CAD build for the part. Positions are in the model's coordinates, mm. A direction names the side the tool comes from. Round coordinates to 2 decimals unless told otherwise and drop trailing zeros. Write each loop counter-clockwise with the first axis right and the second up, starting at its lowest first coordinate (ties: lowest second). Pieces come first, ordered by that corner, then holes. Notation, with made-up numbers: (2, -3.75) - (23, -3.75) arc R17 cw to (23, 1.25) - close; hole circle Ø11 at (63.5, 84). An arc over 180 degrees is marked (long way). Put each result on its own line as item: value. Start each with the question number.
Item 1: Cut at B-B (z = 37). Give the cut face in (x, y).
Item 2: 3-axis set-ups, long thin cutter, end or side, ignore diameter. For faces 1 (the flat face through (127, 3, 44.45)), 2 (the flat face through (-47.625, 3, 130)), 3 (the flat face through (130, 3, -63)), 4 (the flat face through (-79.375, 3, -130)), 5 (the flat face through (63, 3, -133)): which of +Z, -Z, +X, -X, +Y, -Y reach the whole face in a straight line?
Item 3: Pin check, flat tip, straight feed: pin 1 Ø1.5 at (y, z) = (5, -35) entering from +X. Stop position of the tip, or through.
Item 4: Cut at A-A (x = -27). Give the cut face in (y, z), and give its area (3 significant figures).
Item 5: Mould opens along X. For faces 6 (the flat face through (-111.125, 3, -130)), 7 (the flat face through (124, 3, -95)), 8 (the flat face through (32, 3, 127)), 9 (the flat face through (120, 3, -133)) say: released by +X, released by -X, zero draft, split by the parting line, or undercut.
Item 6: Drill centre lines: line 1 (X direction, y = 1.05, z = 32); line 2 (Z direction, x = -43.5, y = 1.2). Where is each one in solid material? Low to high. Write a range as from..to.
```python
from build123d import *

# Parameters (mm, degrees)
SKETCH1_W           = 260
SKETCH1_H           = 266
BOSS_EXTRUDE1_DEPTH = 6
SKETCH2_W           = 31.75
SKETCH2_H           = 6
SKETCH2_W_2         = 6
SKETCH2_H_2         = 25.4
TAB_CUT_OUTS_DEPTH  = 6


with BuildPart() as part:
    # Sketch1 → Boss-Extrude1 (new body)
    with BuildSketch(Plane(origin=(0, 0, 0), x_dir=(1, 0, 0), z_dir=(0, 1, 0))):
        Rectangle(SKETCH1_W, SKETCH1_H)
    extrude(amount=BOSS_EXTRUDE1_DEPTH)

    # Sketch2 → Tab Cut Outs (cut)
    with BuildSketch(Plane(origin=(0, 6, 0), x_dir=(1, 0, 0), z_dir=(0, 1, 0))):
        with Locations((95.25, 130)):
            Rectangle(SKETCH2_W, SKETCH2_H)
        with Locations((-31.75, 130)):
            Rectangle(SKETCH2_W, SKETCH2_H)
        with Locations((-95.25, 130)):
            Rectangle(SKETCH2_W, SKETCH2_H)
        with Locations((31.75, 130)):
            Rectangle(SKETCH2_W, SKETCH2_H)
        with Locations((31.75, -130)):
            Rectangle(SKETCH2_W, SKETCH2_H)
        with Locations((95.25, -130)):
            Rectangle(SKETCH2_W, SKETCH2_H)
        with Locations((-95.25, -130)):
            Rectangle(SKETCH2_W, SKETCH2_H)
        with Locations((-31.75, -130)):
            Rectangle(SKETCH2_W, SKETCH2_H)
        with Locations((127, -95.25)):
            Rectangle(SKETCH2_W_2, SKETCH2_H_2)
        with Locations((127, 31.75)):
            Rectangle(SKETCH2_W_2, SKETCH2_H_2)
        with Locations((127, 95.25)):
            Rectangle(SKETCH2_W_2, SKETCH2_H_2)
        with Locations((127, -31.75)):
            Rectangle(SKETCH2_W_2, SKETCH2_H_2)
    extrude(amount=-TAB_CUT_OUTS_DEPTH, mode=Mode.SUBTRACT)


solid = part.part
```
Output values:
1. outline: (-130, 0) - (124, 0) - (124, 6) - (-130, 6) - close
2. face 1: +X, +Y, -Y
2. face 2: +Z, +Y, -Y
2. face 3: +Z, -Z, +X, +Y, -Y
2. face 4: -Z, +Y, -Y
2. face 5: -Z, +X, -X, +Y, -Y
3. pin 1: x = 124
4. outline: (0, -127) - (6, -127) - (6, 127) - (0, 127) - close
4. area: 1,520 mm2
5. face 6: undercut
5. face 7: released by +X
5. face 8: undercut
5. face 9: zero draft
6. line 1: -130..124
6. line 2: -127..127
